Input: dimensioned drawing with shaded views. Units: mm. Origin: part minimum x, y, z. Coordinates: 2 decimals unless noted, no trailing zeros. Order: outer loops, then holes, each group sorted by start corner. A loop starts at its lowest first (then second) coordinate and runs counter-clockwise, first axis right, second up. Notation, with made-up numbers: M -24,-31 L -15,-31 A14 ccw -15,-23 Z; hole C 51.25,-17.75 d8. An arc over 180 degrees is marked long. Write item = value, one per line.
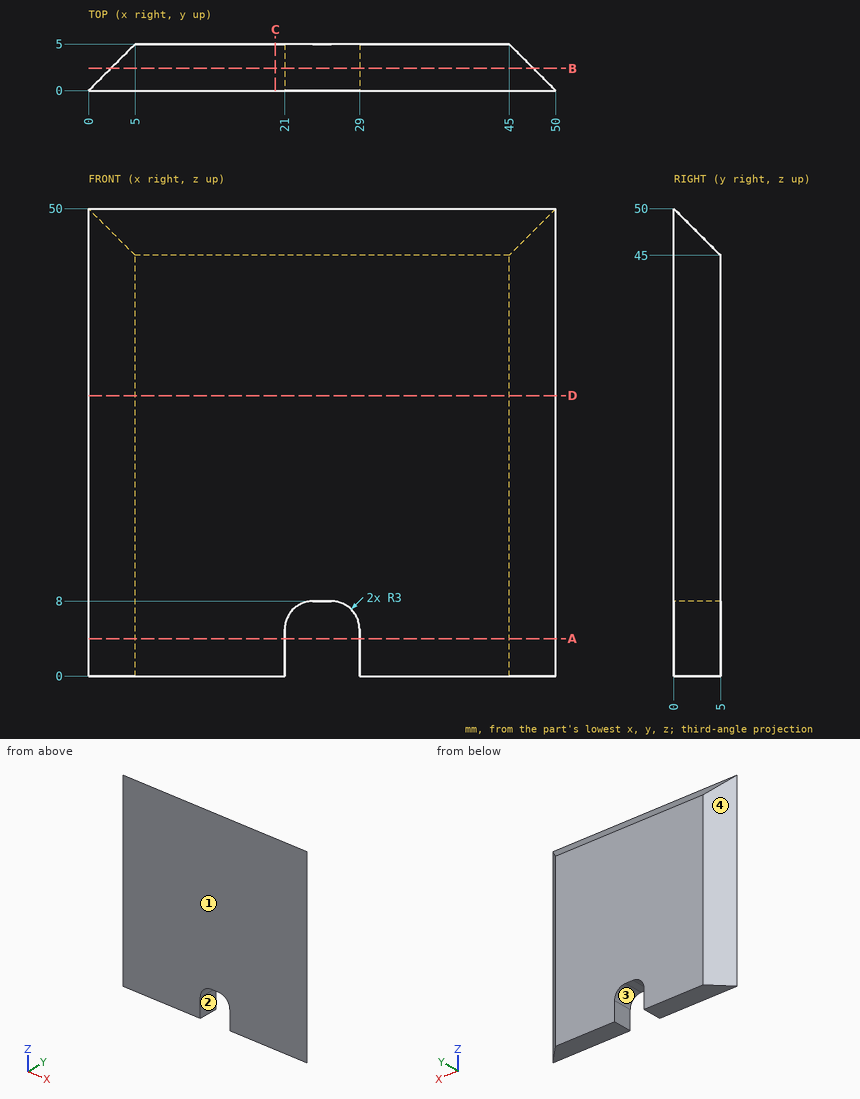
1) Mould query, pull axis X, two halves, no side actions, for the marked faces 1, 2, 3 and 4. Classes: pulls with the +X half, pulls with the -X half, needs draft (parallel to the pull), parting line crosses it, or undercut.
Numbers:
face_1 = needs draft
face_2 = undercut
face_3 = undercut
face_4 = pulls with the -X half
2) Section A-A, the plane z = 4. Return loops of the section in (x, y), and give its area (3 significant figures).
Numbers:
outline = M 0,0 L 21,0 L 21,5 L 5,5 Z; M 29,0 L 50,0 L 45,5 L 29,5 Z
area = 185 mm²
3) Section D-D, the plane z = 30. Return loops of the section in (x, y), and give its area (3 significant figures).
Numbers:
outline = M 0,0 L 50,0 L 45,5 L 5,5 Z
area = 225 mm²
4) Pin query (flat end, axial travel): pin 1 (3 mm diameter, centred on x = 6.5, y = 0.5, fed in from -Z); pin 2 (2 mm diameter, centred on y = 3, z = 25.5, fed in from +X); pin 3 (2 mm diameter, centred on x = 25, y = 3.5, fed in from -Z); pin 4 (1.5 mm diameter, centred on x = 20, y = 3, fed in from +Z). Return the tip coordinate at first contact, or that it passes through.
Numbers:
pin_1 = 0
pin_2 = 48
pin_3 = 8
pin_4 = 47.75
5) Section C-C, the plane x = 20. Return loops of the section in (y, z).
Numbers:
outline = M 0,0 L 5,0 L 5,45 L 0,50 Z
6) Section B-B, the plane y = 2.4. Return loops of the section in (x, z).
Numbers:
outline = M 2.4,0 L 21,0 L 21,5 A3 cw 24,8 L 26,8 A3 cw 29,5 L 29,0 L 47.6,0 L 47.6,47.6 L 2.4,47.6 Z
7) Line query: L1, parallel to Z at x = 11, y = 1.25; L2, parallel to X at y = 1.4, z = 14; L3, parallel to X at y = 4.2, z = 6. Output: solid intervals per line, ascending.
Numbers:
L1 = 0 to 48.75
L2 = 1.4 to 48.6
L3 = 4.2 to 21.17, 28.83 to 45.8
